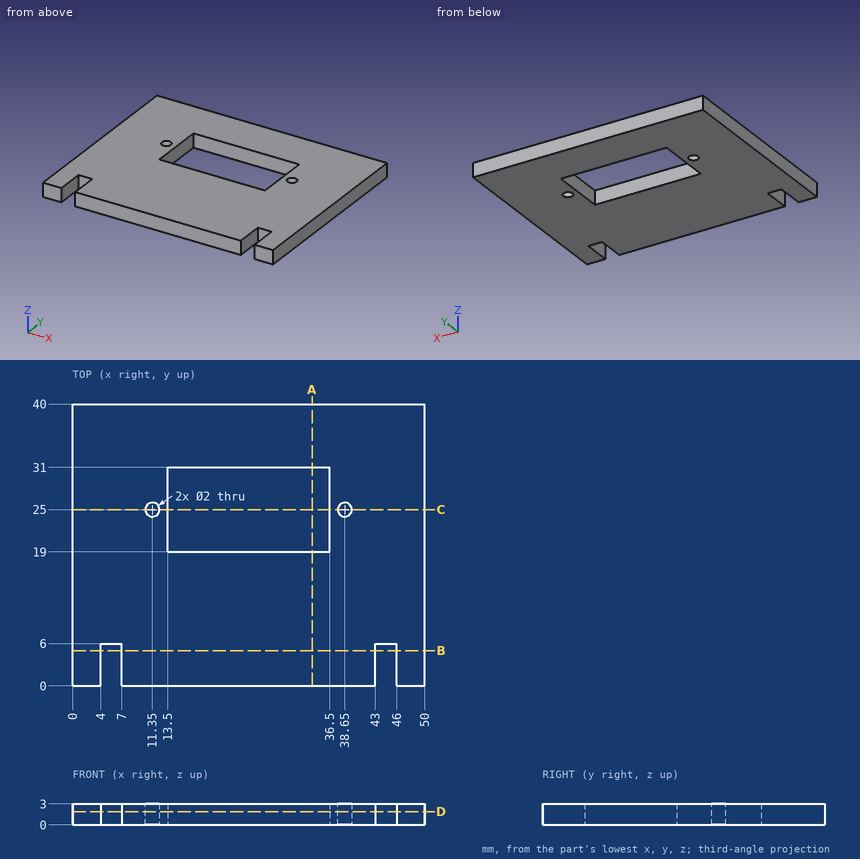
Could you check a few things on this drawing? It's one solid part, dimensions in mm from its lowest x, y, z. Give positions to 0.01 mm unless a question says otherwise; leave off trailing zeros. Loops run counter-clockwise (first coordinate to the right, second up) from the corner with the lowest first, then second, coordinate; pieces in that order, holes last. Notation, with made-up numbers: M -37,16 L -11,16 A20 cw -11,46 Z; hole C 62.25,82.5 d10. An arc over 180 degrees is marked long. Answer as a JSON object with one key per item and string values.
Q1. If I drill on probe 1 along X at (y, z) = (5, 2.35); probe 2 along Y at (x, z) = (38.65, 1.5); probe 3 along Y at (x, z) = (14.5, 1.6), over which ranges is the centre line in solid material (lowest first)? Write a range as [from, to].
Values found:
{"probe 1": "x = [0, 4], [7, 43], [46, 50]", "probe 2": "y = [0, 24], [26, 40]", "probe 3": "y = [0, 19], [31, 40]"}
Q2. Suppose I cut it at B-B, the plane y = 5. List the corners of the cut face in (x, z) for me, plus the area to 3 significant figures.
Values found:
{"outline": "M 0,0 L 4,0 L 4,3 L 0,3 Z; M 7,0 L 43,0 L 43,3 L 7,3 Z; M 46,0 L 50,0 L 50,3 L 46,3 Z", "area": "132 mm²"}
Q3. Suppose I cut it at C-C, the plane y = 25. List the corners of the cut face in (x, z) for me.
Values found:
{"outline": "M 0,0 L 10.35,0 L 10.35,3 L 0,3 Z; M 12.35,0 L 13.5,0 L 13.5,3 L 12.35,3 Z; M 36.5,0 L 37.65,0 L 37.65,3 L 36.5,3 Z; M 39.65,0 L 50,0 L 50,3 L 39.65,3 Z"}
Q4. Suppose I cut it at A-A, the plane x = 34. List the corners of the cut face in (y, z) for me, plus the area to 3 significant figures.
Values found:
{"outline": "M 0,0 L 19,0 L 19,3 L 0,3 Z; M 31,0 L 40,0 L 40,3 L 31,3 Z", "area": "84.0 mm²"}
Q5. Suppose I cut it at D-D, the plane z = 1.9. List the corners of the cut face in (x, y) for me.
Values found:
{"outline": "M 0,0 L 4,0 L 4,6 L 7,6 L 7,0 L 43,0 L 43,6 L 46,6 L 46,0 L 50,0 L 50,40 L 0,40 Z; hole C 11.35,25 d2; hole M 13.5,19 L 36.5,19 L 36.5,31 L 13.5,31 Z; hole C 38.65,25 d2"}
Q6. For P1, Ø1.8, axis at x = 11.35, y = 25, coming from the -Z side; P2, Ø0.9, axis at x = 45, z = 1.5, coming from the -Y side, each with a flat end and sliding along its axis, tell me the tip position at first contact or that it passes through.
Values found:
{"P1": "passes through", "P2": "stops at y = 6"}
